```python
from build123d import *

# Parameters (mm, degrees)
SKETCH1_W           = 60
SKETCH1_H           = 150
BRIDGEPLATE_DEPTH   = 14
SKETCH9_W           = 9
SKETCH9_H           = 6
SKETCH9_H_2         = 5
STRINGNOTCHES_DEPTH = 154.609895515
SKETCH10_W          = 76
SKETCH10_H          = 12
BRIDGEFOOT_DEPTH    = 22


with BuildPart() as part:
    # Sketch1 → BridgePlate (new body)
    with BuildSketch(Plane.XY):
        with Locations((0, 75)):
            Rectangle(SKETCH1_W, SKETCH1_H)
    extrude(amount=BRIDGEPLATE_DEPTH)

    # Sketch9 → StringNotches (cut, through all)
    with BuildSketch(Plane.XY.offset(14)):
        with Locations((-28.5, 30)):
            Rectangle(SKETCH9_W, SKETCH9_H)
        with Locations((-28.5, 41)):
            Rectangle(SKETCH9_W, SKETCH9_H)
        with Locations((-28.5, 52)):
            Rectangle(SKETCH9_W, SKETCH9_H)
        with Locations((-28.5, 63)):
            Rectangle(SKETCH9_W, SKETCH9_H)
        with Locations((-28.5, 74)):
            Rectangle(SKETCH9_W, SKETCH9_H)
        with Locations((-28.5, 85)):
            Rectangle(SKETCH9_W, SKETCH9_H)
        with Locations((-28.5, 96)):
            Rectangle(SKETCH9_W, SKETCH9_H)
        with Locations((-28.5, 107)):
            Rectangle(SKETCH9_W, SKETCH9_H)
        with Locations((-28.5, 118)):
            Rectangle(SKETCH9_W, SKETCH9_H)
        with Locations((-28.5, 129)):
            Rectangle(SKETCH9_W, SKETCH9_H)
        with Locations((-28.5, 140)):
            Rectangle(SKETCH9_W, SKETCH9_H)
        with Locations((28.5, 35.5)):
            Rectangle(SKETCH9_W, SKETCH9_H_2)
        with Locations((28.5, 46.5)):
            Rectangle(SKETCH9_W, SKETCH9_H_2)
        with Locations((28.5, 57.5)):
            Rectangle(SKETCH9_W, SKETCH9_H_2)
        with Locations((28.5, 68.5)):
            Rectangle(SKETCH9_W, SKETCH9_H_2)
        with Locations((28.5, 79.5)):
            Rectangle(SKETCH9_W, SKETCH9_H_2)
        with Locations((28.5, 90.5)):
            Rectangle(SKETCH9_W, SKETCH9_H_2)
        with Locations((28.5, 101.5)):
            Rectangle(SKETCH9_W, SKETCH9_H_2)
        with Locations((28.5, 112.5)):
            Rectangle(SKETCH9_W, SKETCH9_H_2)
        with Locations((28.5, 123.5)):
            Rectangle(SKETCH9_W, SKETCH9_H_2)
        with Locations((28.5, 134.5)):
            Rectangle(SKETCH9_W, SKETCH9_H_2)
    extrude(amount=-STRINGNOTCHES_DEPTH, mode=Mode.SUBTRACT)

    # Sketch10 → BridgeFoot (add)
    with BuildSketch(Plane.XY):
        with Locations((0, 6)):
            Rectangle(SKETCH10_W, SKETCH10_H)
    extrude(amount=BRIDGEFOOT_DEPTH)


solid = part.part
```
Input: part model. Units: mm. Frame: model coordinates. A direction names the side the tool comes from. Round coordinates to 2 decimals unless told otherwise and drop trailing zeros. Loops run counter-clockwise (first coordinate to the right, second up) from the corner with the lowest first, then second, coordinate; pieces in that order, holes last. Notation, with made-up numbers: M 3,-14 L 42,-14 A36 ccw 42,21 Z; hole C 5.5,82 d2. An arc over 180 degrees is marked long. Answer in a Markdown table with one row per item. Add a question column.
1. Section B-B (x = -1). Output: boundary loops of the cut face in (y, z).
2. Ray query, probe 1 along Y at (x, z) = (30, 17.5); probe 2 along X at (y, z) = (81, 1.5); probe 3 along Z at (x, y) = (-23.5, 136). Return the intervals inside material, ascending.
3. Section D-D (z = 17.5). Output: boundary loops of the cut face in (x, y).
4. Section C-C (y = 72.5). Output: boundary loops of the cut face in (x, z), and give its area (3 significant figures).
5. Contact query for flat-ended pins moving along their axis: pin 1 (5 mm diameter, centred on y = 91, z = 5, fed in from -X); pin 2 (10 mm diameter, centred on x = 11.5, y = 62, fed in from +Z); pin 3 (3 mm diameter, centred on x = -26.5, z = 17.5, fed in from +Y). Output: stop coordinate, or through.
6. Mould query, pull axis Y, two halves, no side actions, for faces 1 (the face through (0, 150, 7)), 2 (the face through (-30, 79, 7)), 3 (the face through (27, 93, 7)). Classes: released by +Y, released by -Y, zero draft, split by the parting line, or undercut.
7. Section A-A (x = -26). Give the number of separate pieces and of enclosed holes in the cut face, and give its area (3 significant figures).
8. Set-up query: faces 4 (the face through (30, 85, 7)), 5 (the face through (-30, 35, 7)), 6 (the face through (27, 99, 7)), 7 (the face through (-24, 118, 7)). Return all of +Z, -Z, +X, -X, +Y, -Y with unobstructed straight access to the full face (end or side cutting, diameter ignored); none if empty.
Values follow:
| question | item | result |
|---|---|---|
| 1 | outline | M 0,0 L 150,0 L 150,14 L 12,14 L 12,22 L 0,22 Z |
| 2 | probe 1 | 0 to 12 |
| 2 | probe 2 | -30 to 24 |
| 2 | probe 3 | 0 to 14 |
| 3 | outline | M -38,0 L 38,0 L 38,12 L -38,12 Z |
| 4 | outline | M -24,0 L 30,0 L 30,14 L -24,14 Z |
| 4 | area | 756 mm^2 |
| 5 | pin 1 | x = -30 |
| 5 | pin 2 | z = 14 |
| 5 | pin 3 | y = 12 |
| 6 | face 1 | released by +Y |
| 6 | face 2 | zero draft |
| 6 | face 3 | undercut |
| 7 | separate pieces | 12 |
| 7 | enclosed holes | 0 |
| 7 | area | 1,270 mm^2 |
| 8 | face 4 | +Z, -Z, +X, +Y |
| 8 | face 5 | +Z, -Z, -X, +Y |
| 8 | face 6 | +Z, -Z, +X |
| 8 | face 7 | +Z, -Z, -X |
